```python
from build123d import *

# Parameters (mm, degrees)
SKETCH1_R           = 3
BOSS_EXTRUDE1_DEPTH = 30
SKETCH2_R           = 5.8
BOSS_EXTRUDE2_DEPTH = 4.3
FILLET1_R           = 1


with BuildPart() as part:
    # Sketch1 → Boss-Extrude1 (new body)
    with BuildSketch(Plane(origin=(0, 0, 0), x_dir=(1, 0, 0), z_dir=(0, 1, 0))):
        with Locations(Location((0, 0, 0), (0, 0, 270))):  # turned: the seam where the file's is
            Circle(SKETCH1_R)
    extrude(amount=BOSS_EXTRUDE1_DEPTH)

    # Sketch2 → Boss-Extrude2 (add)
    with BuildSketch(Plane(origin=(0, 30, 0), x_dir=(1, 0, 0), z_dir=(0, 1, 0))):
        with Locations(Location((0, 0, 0), (0, 0, 270))):  # turned: the seam where the file's is
            Circle(SKETCH2_R)
    extrude(amount=BOSS_EXTRUDE2_DEPTH)

    # Fillet1
    fillet1_edges = [part.edges().sort_by_distance(p)[0] for p in [
        (0, 30, -5.8),
        (0, 34.3, -5.8),
    ]]
    fillet(fillet1_edges, radius=FILLET1_R)


solid = part.part
```
Could you check a few things on this model? Use its own coordinates, in mm. A direction names the side the tool comes from. Round coordinates to 2 decimals unless told otherwise and drop trailing zeros. Write each loop counter-clockwise with the first axis right and the second up, starting at its lowest first coordinate (ties: lowest second). Pieces come first, ordered by that corner, then holes. Notation, with made-up numbers: M 86,-22.5 L 142,-22.5 A30 ccw 142,9.5 Z; hole C -8.5,-37.5 d1. An arc over 180 degrees is marked long. Write each question's results on one line, items separated by ' | '. Start each with the question number.
1. Imagine slicing it at C-C on y = 23. List the corners of the cut face in (x, z) for me.
2. I'm going to push flat-ended pins straight in: pin 1 Ø5 at (y, z) = (18.5, -1) entering from -X; pin 2 Ø5 at (x, y) = (0.5, 19.5) entering from -Z; pin 3 Ø2 at (x, y) = (2, 25) entering from +Z. Where does each tip first touch, or does it pass through?
3. I need wall thicknesses on L1, parallel to Y at x = 1.75, z = -4.5; L2, parallel to X at y = 14, z = 0; L3, parallel to Z at x = -1.25, y = 8. Which ranges of each line are inside material? Lowest first, please. Write a range as from..to.
4. Imagine slicing it at A-A on x = 0. List the corners of the cut face in (y, z) for me, and give its area (3 significant figures).
5. Imagine slicing it at B-B on z = 0. List the corners of the cut face in (x, y) for me, and give its area (3 significant figures).
6. On a 3-axis mill with a long thin cutter (end or side, diameter ignored), from which of +Z, -Z, +X, -X, +Y, -Y can I reach the whole of each face in a straight line? I mean faces 1 (the face through (-3, 30, 1)), 2 (the face through (0, 34.3, 0)). Say none if no direction works.
Result sheet:
1) outline: C 0,0 d6
2) pin 1: stops at x = -3 | pin 2: stops at z = -3 | pin 3: stops at z = 2.83
3) L1: y = 30..34.3 | L2: x = -3..3 | L3: z = -2.73..2.73
4) outline: M 0,-3 L 30,-3 L 30,-4.8 A1 ccw 31,-5.8 L 33.3,-5.8 A1 ccw 34.3,-4.8 L 34.3,4.8 A1 ccw 33.3,5.8 L 31,5.8 A1 ccw 30,4.8 L 30,3 L 0,3 Z | area: 229 mm^2
5) outline: M -5.8,31 A1 ccw -4.8,30 L -3,30 L -3,0 L 3,0 L 3,30 L 4.8,30 A1 ccw 5.8,31 L 5.8,33.3 A1 ccw 4.8,34.3 L -4.8,34.3 A1 ccw -5.8,33.3 Z | area: 229 mm^2
6) face 1: -Y | face 2: +Z, -Z, +X, -X, +Y
